Source: CAD feature listing. Evaluate the final solid. Frame: model axes, mm. Face numbers are marked on the shaded views. A direction names the side the tool comes from. Give positions to 0.01 mm unless a question says otherwise; leave off trailing zeros. Loops run counter-clockwise (first coordinate to the right, second up) from the corner with the lowest first, then second, coordinate; pieces in that order, holes last. Notation, with made-up numbers: (62.25, 9) - (113.25, 9) arc R19 ccw to (113.25, 18) - close; hole circle Ø9 at (10, 29). An arc over 180 degrees is marked (long way). Put each result on its own line as item: value.
```python
from build123d import *

# Parameters (mm, degrees)
PAD002_DEPTH = 0.3
PAD_DEPTH    = 2.415
CHAMFER_SIZE = 0.5
PAD001_DEPTH = 0.3


with BuildPart() as pad002:
    # Sketch002 → Pad002 (new body, symmetric)
    with BuildSketch(Plane.XZ.offset(2.54)):
        Polygon((-0.2, -3), (0.2, -3), (0.2, 1.08), (4.88, 1.08), (4.88, -3), (5.28, -3), (5.28, 1.48), (-0.2, 1.48), align=None)
    extrude(amount=PAD002_DEPTH, both=True)


with BuildPart() as chamfer_body:
    # Sketch → Pad (new body, symmetric)
    with BuildSketch(Plane.XZ.offset(1.27)):
        Polygon((0.59, 0.2), (4.49, 0.2), (4.59, 1.28), (4.49, 2.9), (0.59, 2.9), (0.49, 1.28), align=None)
    extrude(amount=PAD_DEPTH, both=True)

    # Chamfer
    chamfer_edges = [chamfer_body.edges().sort_by_distance(p)[0] for p in [
        (0.59, -1.27, 2.9),
    ]]
    chamfer(chamfer_edges, length=CHAMFER_SIZE)


with BuildPart() as diode_bridge_dip_4_w5_08mm_p2_54mm:
    # Sketch001 → Pad001 (new body, symmetric)
    with BuildSketch(Plane.XZ):
        Polygon((-0.2, -3), (0.2, -3), (0.2, 1.08), (4.88, 1.08), (4.88, -3), (5.28, -3), (5.28, 1.48), (-0.2, 1.48), align=None)
    extrude(amount=PAD001_DEPTH, both=True)

    add(pad002.part)
    add(chamfer_body.part)


solid = diode_bridge_dip_4_w5_08mm_p2_54mm.part
```
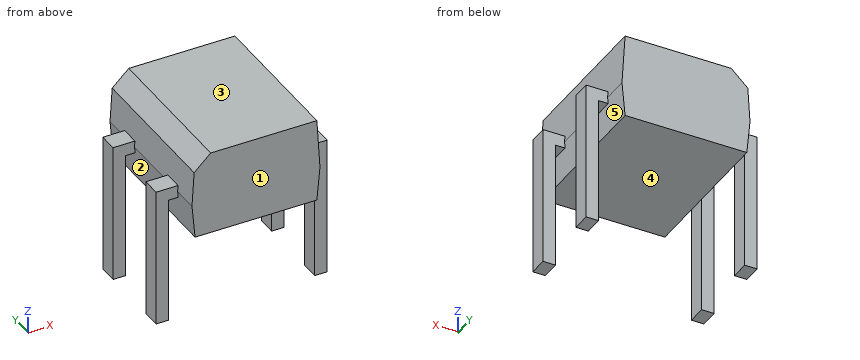
1) Section query D-D, the plane x = 4.3. Output: boundary loops of the cut face in (y, z) (3 decimals).
Check result:
outline: (-3.685, 0.2) - (1.145, 0.2) - (1.145, 2.9) - (-3.685, 2.9) - close
2) Material intervals for line 1 along Y through (x, z) = (0, -1.1); line 2 along X through (y, z) = (-0.15, 1); line 3 along X through (y, z) = (-2.55, -2.2), sorted ascending. Write a range as [from, to].
Check result:
line 1: [-2.84, -2.24], [-0.3, 0.3]
line 2: [-0.2, 0.2], [0.52, 4.56], [4.88, 5.28]
line 3: [-0.2, 0.2], [4.88, 5.28]
3) Pin query (flat end, axial travel): P1, Ø0.8, axis at x = 0, z = 0, coming from the -Y side; P2, Ø0.6, axis at x = 5, z = 0, coming from the +Y side; P3, Ø1, axis at x = 1.5, y = -2.5, coming from the -Z side; P4, Ø2, axis at y = 0.5, z = -1, coming from the +X side. Return the tip coordinate at first contact, or that it passes through.
Check result:
P1: y = -2.84
P2: y = 0.3
P3: z = 0.2
P4: x = 5.28
4) Access query for the marked faces 3, 4 and 5. Directions: +Z, -Z, +X, -X, +Y, -Y. A direction counts if a zero-diameter tool reaches every point of the face in a straight line with its end or side. Return the directions, or none.
Check result:
face 3: +Z, +X, -X, +Y, -Y
face 4: -Z, +Y, -Y
face 5: -Z
5) Section query C-C, the plane z = 0.6. Output: boundary loops of the cut face in (x, y) (3 decimals).
Check result:
outline: (-0.2, -2.84) - (0.2, -2.84) - (0.2, -2.24) - (-0.2, -2.24) - close; (-0.2, -0.3) - (0.2, -0.3) - (0.2, 0.3) - (-0.2, 0.3) - close; (0.553, -3.685) - (4.527, -3.685) - (4.527, 1.145) - (0.553, 1.145) - close; (4.88, -2.84) - (5.28, -2.84) - (5.28, -2.24) - (4.88, -2.24) - close; (4.88, -0.3) - (5.28, -0.3) - (5.28, 0.3) - (4.88, 0.3) - close
6) Section query B-B, the plane y = -1.3. Output: boundary loops of the cut face in (x, z), plus the area to 3 significant figures.
Check result:
outline: (0.49, 1.28) - (0.59, 0.2) - (4.49, 0.2) - (4.59, 1.28) - (4.49, 2.9) - (1.09, 2.9) - (0.56, 2.4) - close
area: 10.7 mm²
7) Section query A-A, the plane z = -2.25. Output: boundary loops of the cut face in (x, y), plus the area to 3 significant figures.
Check result:
outline: (-0.2, -2.84) - (0.2, -2.84) - (0.2, -2.24) - (-0.2, -2.24) - close; (-0.2, -0.3) - (0.2, -0.3) - (0.2, 0.3) - (-0.2, 0.3) - close; (4.88, -2.84) - (5.28, -2.84) - (5.28, -2.24) - (4.88, -2.24) - close; (4.88, -0.3) - (5.28, -0.3) - (5.28, 0.3) - (4.88, 0.3) - close
area: 0.960 mm²
8) Mould query, pull axis X, two halves, no side actions, for the marked faces 1 and 2. Classes: pulls with the +X half, pulls with the -X half, needs draft (parallel to the pull), parting line crosses it, or undercut.
Check result:
face 1: needs draft
face 2: undercut
